Could you check a few things on this model? Use its own coordinates, in mm. A direction names the side the tool comes from. Round coordinates to 2 decimals unless told otherwise and drop trailing zeros. Loops run counter-clockwise (first coordinate to the right, second up) from the corner with the lowest first, then second, coordinate; pieces in that order, holes last. Notation, with made-up numbers: M 46,67 L 63,67 A15 cw 63,74 Z; hole C 1,14 d6. An arc over 180 degrees is marked long. Answer in a Markdown table with one row per item.
```python
from build123d import *

# Parameters (mm, degrees)
SKETCH1_R           = 3
BOSS_EXTRUDE1_DEPTH = 7
BOSS_EXTRUDE2_DEPTH = 20
FILLET1_R           = 0.75


with BuildPart() as part:
    # Sketch1 → Boss-Extrude1 (new body)
    with BuildSketch(Plane(origin=(0, 0, 0), x_dir=(1, 0, 0), z_dir=(0, 1, 0))):
        with BuildLine():
            Line((-55, 10), (55, 10))
            ThreePointArc((55, 10), (65, 0), (55, -10))
            Line((55, -10), (-55, -10))
            ThreePointArc((-55, -10), (-65, 0), (-55, 10))
        make_face()
        with Locations(Location((-55, 0, 0), (0, 0, 270))):
            Circle(SKETCH1_R, mode=Mode.SUBTRACT)
        with Locations(Location((55, 0, 0), (0, 0, 270))):
            Circle(SKETCH1_R, mode=Mode.SUBTRACT)
    extrude(amount=BOSS_EXTRUDE1_DEPTH)

    # Sketch2 → Boss-Extrude2 (add)
    with BuildSketch(Plane.XY.offset(10)):
        with BuildLine():
            Line((-9.5e-08, 7), (36, 7))
            Line((36, 7), (36, 34))
            ThreePointArc((36, 34), (22.499999962, 14.499999972), (-9.5e-08, 7))
        make_face()
        with BuildLine():
            Line((-36, 7), (-9.5e-08, 7))
            ThreePointArc((-9.5e-08, 7), (-22.500000038, 14.500000028), (-36, 34))
            Line((-36, 34), (-36, 7))
        make_face()
    extrude(amount=-BOSS_EXTRUDE2_DEPTH)

    # Fillet1
    fillet1_edges = [part.edges().sort_by_distance(p)[0] for p in [
        (65, 7, 0),
        (45.5, 7, -10),
        (45.5, 7, 10),
        (36, 20.5, 10),
        (36, 34, 0),
        (0, 7, -10),
        (0, 7, 10),
        (36, 20.5, -10),
        (-45.5, 7, -10),
        (-36, 20.5, -10),
        (-36, 20.5, 10),
        (-36, 34, 0),
        (-65, 7, 0),
        (-45.5, 7, 10),
    ]]
    fillet(fillet1_edges, radius=FILLET1_R)


solid = part.part
```
1) I want a section at A-A, the plane z = 0. Please give me the cut outline in (x, y).
Computed:
| item | result |
|---|---|
| outline | M -65,0 L -58,0 L -58,7 L -64.25,7 A0.75 ccw -65,6.25 Z; M -52,0 L 52,0 L 52,7 L 36,7 L 36,29.65 A0.75 ccw 34.56,29.94 A37.5 cw -34.56,29.94 A0.75 ccw -36,29.65 L -36,7 L -52,7 Z; M 58,0 L 65,0 L 65,6.25 A0.75 ccw 64.25,7 L 58,7 Z |
2) I want a section at B-B, the plane y = 4. Please give me the cut outline in (x, z).
Computed:
| item | result |
|---|---|
| outline | M -55,-10 L 55,-10 A10 ccw 55,10 L -55,10 A10 ccw Z; hole C -55,0 d6; hole C 55,0 d6 |
3) I need wall thicknesses on line 1 (X direction, y = 4, z = 0); line 2 (Y direction, x = -39.5, z = 2.5); line 3 (X direction, y = 6.5, z = 2.5). Which ranges of each line are inside material? Lowest first, please.
Computed:
| item | result |
|---|---|
| line 1 | x = -65 to -58, -52 to 52, 58 to 65 |
| line 2 | y = 0 to 7 |
| line 3 | x = -64.64 to -56.66, -53.34 to 53.34, 56.66 to 64.64 |
4) If we mould it in two halves opening along X, with no side actions, what happens to faces 1 (the face through (58, 3, 0)), 2 (the face through (-52, 3, 0)), 3 (the face through (0, 5, 10)), 4 (the face through (-65, 3, 0))? For each: released by +X, released by -X, zero draft, split by the parting line, or undercut.
Computed:
| item | result |
|---|---|
| face 1 | undercut |
| face 2 | undercut |
| face 3 | zero draft |
| face 4 | released by -X |
5) Will these pins go through, and if not, where does the flat tip stop? P1, Ø8, axis at x = -9.5, z = 0.5, coming from the +Y side; P2, Ø6, axis at x = 29, z = 1.5, coming from the -Y side; P3, Ø3.5, axis at x = -55, z = 0, coming from the +Y side; P4, Ø5.5, axis at x = 47.5, z = -1.5, coming from the +Y side.
Computed:
| item | result |
|---|---|
| P1 | stops at y = 9.51 |
| P2 | stops at y = 0 |
| P3 | passes through |
| P4 | stops at y = 7 |
6) Which directions (+Z, -Z, +X, -X, +Y, -Y) give clear straight access to the entire face, cutting with the end or side of a thin tool? Please do faces 5 (the face through (-36, 18, 0)), 6 (the face through (0, 5, -10)), 7 (the face through (50, 7, 0)).
Computed:
| item | result |
|---|---|
| face 5 | +Z, -Z, -X, +Y |
| face 6 | -Z, +X, -X, +Y, -Y |
| face 7 | +Z, -Z, +X, +Y |
